Part model, mm, in its own coordinate system. A direction names the side the tool comes from. Round coordinates to 2 decimals unless told otherwise and drop trailing zeros. Loops run counter-clockwise (first coordinate to the right, second up) from the corner with the lowest first, then second, coordinate; pieces in that order, holes last. Notation, with made-up numbers: M 1.25,82 L 39.25,82 A18 cw 39.25,105 Z; hole C -8,39 d11. An arc over 180 degrees is marked long. Answer as CSV lines item,"result". Start each with the question number.
Item 1: Mould opens along X. For faces 1 (the flat face through (-12, 0, 2.5)), 2 (the cylindrical face through (-27.694, 2.36, 14.79)), 3 (the flat face through (-17, 19, 0)) say: pulls with the +X half, pulls with the -X half, needs draft (parallel to the pull), parting line crosses it, or undercut.
Item 2: Drop flat-ended pins along their axis: pin 1 Ø1.5 at (y, z) = (27.5, 13) entering from +X; pin 2 Ø1.5 at (x, z) = (-26.5, 13) entering from -Y; pin 3 Ø5 at (y, z) = (-0.5, 9.5) entering from +X. Give the stop position or say it passes through.
Item 3: Which spindle directions (+Z, -Z, +X, -X, +Y, -Y) get a long thin tool onto all of the face, cutting with end or side? Do faces 4 (the flat face through (-8.648, 0, 16)), 5 (the flat face through (-8, 15, 30)), 6 (the cylindrical face through (-10.63, 9.16, 0.25)). Say none if no direction does.
Item 4: Band-saw the part on D-D (x = -2.5). Give the cut face in (y, z), and give its area (3 significant figures).
Item 5: Band-saw the part on B-B (x = -27.5). Give the cut face in (y, z).
Item 6: Band-saw the part on A-A (z = 13.5). Give the cut face in (x, y), and give its area (3 significant figures).
Item 7: Band-saw the part on C-C (y = -2). Give the cut face in (x, z), and give its area (3 significant figures).
Item 8: Wall check: line 1 (X direction, y = 14.5, z = 5.75); line 2 (X direction, y = 16.5, z = 14.25); line 3 (Y direction, x = -11.5, z = 15.25). Give the ranges that are in metal, low to high.
```python
from build123d import *

# Parameters (mm, degrees)
SKETCH1_R                       = 20
SKETCH1_R_2                     = 1
BOSS_EXTRUDE1_DEPTH             = 30
TAP_DRILL_FOR_M5X0_8_TAP1_D     = 4.2
TAP_DRILL_FOR_M5X0_8_TAP1_DEPTH = 5
TAP_DRILL_FOR_M5X0_8_TAP1_TIP   = 1.2618073
SKETCH4_W                       = 6.5
SKETCH4_H                       = 6.5
CUT_EXTRUDE1_DEPTH              = 27.5
CIRPATTERN1_COUNT               = 4
SKETCH5_R                       = 6.5
SKETCH5_R_2                     = 5.5
CUT_EXTRUDE2_DEPTH              = 1
FILLET3_R                       = 0.5


with BuildPart() as part:
    # Sketch1 → Boss-Extrude1 (new body)
    with BuildSketch(Plane.XY):
        with Locations((-11.822558412, 14.529752947)):
            Circle(SKETCH1_R)
        with Locations((-11.822558412, 14.529752947)):
            Circle(SKETCH1_R_2, mode=Mode.SUBTRACT)
    extrude(amount=BOSS_EXTRUDE1_DEPTH)

    # Tap Drill for M5x0.8 Tap1
    with Locations(Plane.XY.offset(30)):
        with Locations((-11.822558412, 14.529752947)):
            Hole(TAP_DRILL_FOR_M5X0_8_TAP1_D / 2, depth=TAP_DRILL_FOR_M5X0_8_TAP1_DEPTH)
            with Locations((0, 0, -(TAP_DRILL_FOR_M5X0_8_TAP1_DEPTH + TAP_DRILL_FOR_M5X0_8_TAP1_TIP / 2))):  # 118° drill point
                Cone(0, TAP_DRILL_FOR_M5X0_8_TAP1_D / 2, TAP_DRILL_FOR_M5X0_8_TAP1_TIP, mode=Mode.SUBTRACT)

    # Sketch4 → Cut-Extrude1 (cut)
    with BuildSketch(Plane.XY.offset(30)):
        with Locations((2.927441588, 14.454752947)):
            Rectangle(SKETCH4_W, SKETCH4_H)
    cut_extrude1 = extrude(amount=-CUT_EXTRUDE1_DEPTH, mode=Mode.SUBTRACT)

    # CirPattern1: Cut-Extrude1 ×4 about axis
    cirpattern1_axis = Axis((-11.822558412, 14.529752947, 0), (0, 0, 1))
    for i in range(1, CIRPATTERN1_COUNT):
        add(cut_extrude1.rotate(cirpattern1_axis, i * 360 / CIRPATTERN1_COUNT), mode=Mode.SUBTRACT)

    # Sketch5 → Cut-Extrude2 (cut)
    with BuildSketch(Plane(origin=(0, 0, 0), x_dir=(-1, 0, 0), z_dir=(0, 0, -1))):
        with Locations((11.822558412, 14.529752947)):
            Circle(SKETCH5_R)
        with Locations((11.822558412, 14.529752947)):
            Circle(SKETCH5_R_2, mode=Mode.SUBTRACT)
    extrude(amount=-CUT_EXTRUDE2_DEPTH, mode=Mode.SUBTRACT)

    # Fillet3
    fillet3_edges = [part.edges().sort_by_distance(p)[0] for p in [
        (-5.322558412, 14.529752947, 1),
        (-6.322558412, 14.529752947, 1),
    ]]
    fillet(fillet3_edges, radius=FILLET3_R - 0.0001)  # a hair under: the kernel refuses the full size


solid = part.part
```
Answer block:
1,face 1,"undercut"
1,face 2,"parting line crosses it"
1,face 3,"needs draft"
2,pin 1,"stops at x = 4.01"
2,pin 2,"stops at y = 0.18"
2,pin 3,"stops at x = 3.77"
3,face 4,"+Z"
3,face 5,"+Z, +X, -X, +Y, -Y"
3,face 6,"-Z"
4,outline,"M -3.16,0 L 32.22,0 L 32.22,30 L -3.16,30 Z"
4,area,"1,060 mm^2"
5,outline,"M 2.11,0 L 26.95,0 L 26.95,30 L 17.85,30 L 17.85,2.5 L 11.35,2.5 L 11.35,30 L 2.11,30 Z"
6,outline,"C -11.82,14.53 d40; hole M -29.82,11.35 L -23.32,11.35 L -23.32,17.85 L -29.82,17.85 Z; hole M -15.15,-3.47 L -8.65,-3.47 L -8.65,3.03 L -15.15,3.03 Z; hole M -15,26.03 L -8.5,26.03 L -8.5,32.53 L -15,32.53 Z; hole C -11.82,14.53 d2; hole M -0.32,11.2 L 6.18,11.2 L 6.18,17.7 L -0.32,17.7 Z"
6,area,"1,080 mm^2"
7,outline,"M -23.08,0 L -0.56,0 L -0.56,30 L -8.65,30 L -8.65,2.5 L -15.15,2.5 L -15.15,30 L -23.08,30 Z"
7,area,"497 mm^2"
8,line 1,"x = -31.82 to -29.82, -23.32 to -12.82, -10.82 to -0.32, 6.18 to 8.18"
8,line 2,"x = -31.73 to -29.82, -23.32 to -0.32, 6.18 to 8.08"
8,line 3,"y = -5.47 to -3.47, 3.03 to 13.58, 15.48 to 26.03, 32.53 to 34.53"
